Work out the finished part from the listing and answer in its coordinate system (mm). A direction names the side the tool comes from. Round coordinates to 2 decimals unless told otherwise and drop trailing zeros. Order: outer loops, then holes, each group sorted by start corner. A loop starts at its lowest first (then second) coordinate and runs counter-clockwise, first axis right, second up. Notation, with made-up numbers: (-3, 16) - (55, 16) arc R14 ccw to (55, 22) - close; hole circle Ø8 at (-6.75, -40). An arc over 180 degrees is marked (long way). Use one line per item in the form item = value. Start each with the question number.
Q1. Which of the six approach directions +Z, -Z, +X, -X, +Y, -Y give full straight-line access (tool end or side, diameter ignored) to faces 1 (the flat face through (-61, 18, 40)), 2 (the flat face through (-40, 17, 1))?
Q2. For a pull along Y with two mould halves and no side action, classify faces 3 (the flat face through (-61, 0, 20)), 4 (the flat face through (-20, 17, 2.5)), 5 (the flat face through (-15, 17, 25)), 6 (the flat face through (-15, 17, 10)) as +Y half, -Y half, draft (parallel to the pull), parting line (faces both ways), or undercut.
Q3. The part is cut by section A-A on y = 6. Determine the outline of the cut face in (x, z), plus the area to 3 significant figures.
Q4. Find the intervals of material crossed by line 1 (Z direction, x = -8.75, y = 17.5); line 2 (Z direction, x = -10.5, y = 19); line 3 (Y direction, x = -4.25, z = 25), in increasing order. Write a range as [from, to].
Q5. Given P1, Ø12, axis at x = -25.5, y = 30, coming from the -Z side; P2, Ø5, axis at x = -100.5, z = 18, coming from the -Y side; P3, Ø1.3, axis at y = 18, z = 25, coming from the +X side, each flat-ended and moving along its own axis, determine where each tip first touches the part or whether it passes through.
from build123d import *

# Parameters (mm, degrees)
F0_W     = 120
F0_H     = 35
F1_DEPTH = 40
F3_DEPTH = 15
F4_W     = 35
F4_H     = 2.5
F5_DEPTH = 40


with BuildPart() as f1:
    # F0 (on Top) → F1 (new body)
    with BuildSketch(Plane.XY):
        with Locations((-60, 17.5)):
            Rectangle(F0_W, F0_H)
    extrude(amount=F1_DEPTH)

    # F2 (on face) → F3 (cut)
    with BuildSketch(Plane.YZ):
        with BuildLine():
            ThreePointArc((17.5, 12.1), (15.4, 10), (17.5, 7.9))
            Line((17.5, 7.9), (17.5, 10))
            Line((17.5, 10), (17.5, 12.1))
        make_face()
        with BuildLine():
            ThreePointArc((19.6, 25), (16.015076, 26.484924), (17.5, 22.9))
            ThreePointArc((17.5, 22.9), (18.984924, 23.515076), (19.6, 25))
        make_face()
        with BuildLine():
            Line((17.5, 10), (17.5, 7.9))
            ThreePointArc((17.5, 7.9), (18.984924, 8.515076), (19.6, 10))
            ThreePointArc((19.6, 10), (18.984924, 11.484924), (17.5, 12.1))
            Line((17.5, 12.1), (17.5, 10))
        make_face()
    extrude(amount=-F3_DEPTH, mode=Mode.SUBTRACT)

    # F4 (on face) → F5 (cut)
    with BuildSketch(Plane.YZ):
        with Locations((17.5, 1.25)):
            Rectangle(F4_W, F4_H)
    extrude(amount=-F5_DEPTH, mode=Mode.SUBTRACT)


solid = f1.part
Found:
q1.face_1 = +Z, +X, -X, +Y, -Y
q1.face_2 = -Z, +X, +Y, -Y
q2.face_3 = -Y half
q2.face_4 = draft
q2.face_5 = undercut
q2.face_6 = undercut
q3.outline = (-120, 0) - (-40, 0) - (-40, 2.5) - (0, 2.5) - (0, 40) - (-120, 40) - close
q3.area = 4,700 mm²
q4.line_1 = [2.5, 7.9], [12.1, 22.9], [27.1, 40]
q4.line_2 = [2.5, 8.53], [11.47, 23.53], [26.47, 40]
q4.line_3 = [0, 15.4], [19.6, 35]
q5.P1 = 2.5
q5.P2 = 0
q5.P3 = -15
